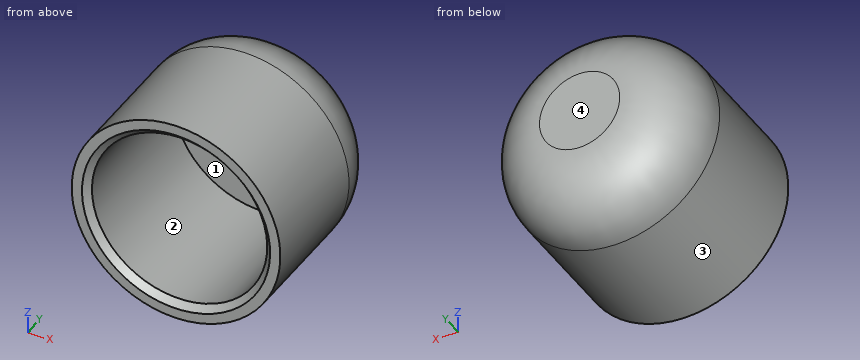
```python
from build123d import *

# Parameters (mm, degrees)
SKETCH1_R           = 16.25
SKETCH1_R_2         = 13.65
BOSS_EXTRUDE1_DEPTH = 24
CHAMFER1_SIZE       = 1
SKETCH3_R           = 16.25
BOSS_EXTRUDE3_DEPTH = 5.2
FILLET3_R           = 10


with BuildPart() as part:
    # Sketch1 → Boss-Extrude1 (new body)
    with BuildSketch(Plane(origin=(0, 0, 0), x_dir=(1, 0, 0), z_dir=(0, 1, 0))):
        with Locations(Location((0, 0, 0), (0, 0, 270))):
            Circle(SKETCH1_R)
        with Locations(Location((0, 0, 0), (0, 0, 270))):
            Circle(SKETCH1_R_2, mode=Mode.SUBTRACT)
    extrude(amount=BOSS_EXTRUDE1_DEPTH)

    # Chamfer1
    chamfer1_edges = [part.edges().sort_by_distance(p)[0] for p in [
        (0, 0, -13.65),
    ]]
    chamfer(chamfer1_edges, length=CHAMFER1_SIZE)

    # Sketch3 → Boss-Extrude3 (add)
    with BuildSketch(Plane(origin=(0, 24, 0), x_dir=(1, 0, 0), z_dir=(0, 1, 0))):
        with Locations(Location((0, 0, 0), (0, 0, 270))):
            Circle(SKETCH3_R)
    extrude(amount=BOSS_EXTRUDE3_DEPTH)

    # Fillet3
    fillet3_edges = [part.edges().sort_by_distance(p)[0] for p in [
        (0, 29.2, -16.25),
    ]]
    fillet(fillet3_edges, radius=FILLET3_R)


solid = part.part
```
Geometry check sheet. Reference: the model listing, model coordinates, mm. Face numbers are marked on the shaded views. Round coordinates to 2 decimals unless told otherwise and drop trailing zeros. Loops run counter-clockwise (first coordinate to the right, second up) from the corner with the lowest first, then second, coordinate; pieces in that order, holes last. Notation, with made-up numbers: (46.5, 36) - (68.5, 36) arc R13 cw to (68.5, 45) - close; hole circle Ø1 at (-5.75, -37). An arc over 180 degrees is marked (long way). Use a Markdown table: item, result.
Q1. Material ranges on line 1 (X direction, y = 12.25, z = 0); line 2 (Z direction, x = 7, y = 20.5); line 3 (X direction, y = 9.25, z = -7) (3 decimals), recorded low to high.
Solutions:
| item | result |
|---|---|
| line 1 | x = -16.25 to -13.65, 13.65 to 16.25 |
| line 2 | z = -14.57 to -11.72, 11.72 to 14.57 |
| line 3 | x = -14.665 to -11.718, 11.718 to 14.665 |
Q2. Go/stop test with flat-tipped pins: P1, Ø1.5, axis at x = -6.5, y = 22, coming from the +Z side; P2, Ø3, axis at x = 2.5, y = 23, coming from the +Z side; P3, Ø1.5, axis at y = 20.5, z = -10, coming from the +X side. Record where each tip stops, or that it passes through.
Solutions:
| item | result |
|---|---|
| P1 | stops at z = 14.84 |
| P2 | stops at z = 15.84 |
| P3 | stops at x = 13.27 |
Q3. Draft check along X on the marked faces 1, 2, 3 and 4. Enter one of: released by +X, released by -X, zero draft, split by the parting line, or undercut.
Solutions:
| item | result |
|---|---|
| face 1 | undercut |
| face 2 | undercut |
| face 3 | split by the parting line |
| face 4 | zero draft |
Q4. Cross-section at A-A on y = 15.5. Record the cut outline in (x, z).
Solutions:
| item | result |
|---|---|
| outline | circle Ø32.5 at (0, 0); hole circle Ø27.3 at (0, 0) |
